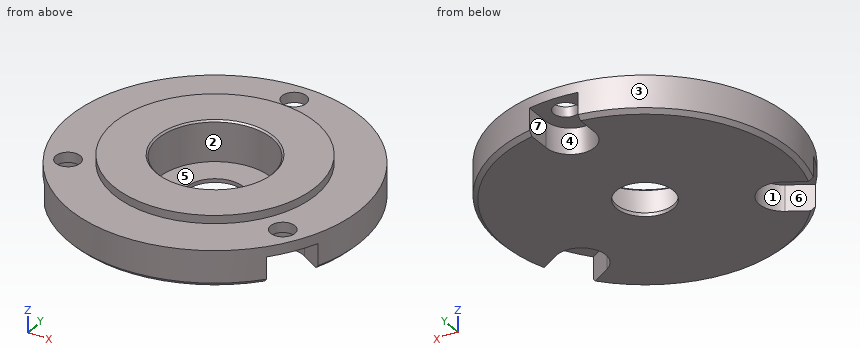
from build123d import *

# Parameters (mm, degrees)
ESQUISSE1_R             = 17.97
BOSS_EXTRU_1_DEPTH      = 4.45
ESQUISSE2_R             = 12.45
BOSS_EXTRU_2_DEPTH      = 1
CHANFREIN1_SIZE         = 0.5
ESQUISSE5_R             = 1.5
ENL_V_MAT_EXTRU_1_DEPTH = 6.45
ESQUISSE6_R             = 3.5
ENL_V_MAT_EXTRU_2_DEPTH = 6.45
ESQUISSE7_R             = 7
ENL_V_MAT_EXTRU_3_DEPTH = 5
ENL_V_MAT_EXTRU_4_DEPTH = 3.2
CHANFREIN2_SIZE         = 0.2


with BuildPart() as part:
    # Esquisse1 → Boss.-Extru.1 (new body)
    with BuildSketch(Plane.XY):
        with Locations((-74.842203198, 51.872077922)):
            Circle(ESQUISSE1_R)
    extrude(amount=BOSS_EXTRU_1_DEPTH)

    # Esquisse2 → Boss.-Extru.2 (add)
    with BuildSketch(Plane.XY.offset(4.45)):
        with Locations((-74.842203198, 51.872077922)):
            Circle(ESQUISSE2_R)
    extrude(amount=BOSS_EXTRU_2_DEPTH)

    # Chanfrein1
    chanfrein1_edges = [part.edges().sort_by_distance(p)[0] for p in [
        (-92.812203198, 51.872077922, 0),
    ]]
    chamfer(chanfrein1_edges, length=CHANFREIN1_SIZE)

    # Esquisse5 → Enlèv. mat.-Extru.1 (cut, through all)
    with BuildSketch(Plane(origin=(0, 0, 0), x_dir=(-1, 0, 0), z_dir=(0, 0, -1))):
        with Locations((74.842203198, 67.242077922)):
            Circle(ESQUISSE5_R)
        with Locations((61.531392742, 44.187077922)):
            Circle(ESQUISSE5_R)
        with Locations((88.153013654, 44.187077922)):
            Circle(ESQUISSE5_R)
    extrude(amount=-ENL_V_MAT_EXTRU_1_DEPTH, mode=Mode.SUBTRACT)

    # Esquisse6 → Enlèv. mat.-Extru.2 (cut, through all)
    with BuildSketch(Plane(origin=(0, 0, 0), x_dir=(-1, 0, 0), z_dir=(0, 0, -1))):
        with Locations((74.842203198, 51.872077922)):
            Circle(ESQUISSE6_R)
    extrude(amount=-ENL_V_MAT_EXTRU_2_DEPTH, mode=Mode.SUBTRACT)

    # Esquisse7 → Enlèv. mat.-Extru.3 (cut)
    with BuildSketch(Plane.XY.offset(5.45)):
        with Locations((-74.842203198, 51.872077922)):
            Circle(ESQUISSE7_R)
    extrude(amount=-ENL_V_MAT_EXTRU_3_DEPTH, mode=Mode.SUBTRACT)

    # Esquisse8 → Enlèv. mat.-Extru.4 (cut)
    with BuildSketch(Plane(origin=(0, 0, 0), x_dir=(-1, 0, 0), z_dir=(0, 0, -1))):
        with BuildLine():
            Line((71.842203198, 70.411905134), (71.842203198, 66.363654544))
            ThreePointArc((71.842203198, 66.363654544), (74.842203198, 63.363654544), (77.842203198, 66.363654544))
            Line((77.842203198, 66.363654544), (77.842203198, 70.411905134))
            Line((77.842203198, 70.411905134), (71.842203198, 70.411905134))
        make_face()
        with BuildLine():
            Line((60.379554388, 39.925212907), (63.849582418, 42.010216097))
            ThreePointArc((63.849582418, 42.010216097), (64.875970095, 46.126832224), (60.759353968, 47.153219901))
            Line((60.759353968, 47.153219901), (57.289325938, 45.068216711))
            Line((57.289325938, 45.068216711), (60.379554388, 39.925212907))
        make_face()
        with BuildLine():
            Line((92.371338943, 45.133431645), (88.865451092, 47.15755694))
            ThreePointArc((88.865451092, 47.15755694), (84.76737488, 46.059480728), (85.865451092, 41.961404517))
            Line((85.865451092, 41.961404517), (89.371338943, 39.937279222))
            Line((89.371338943, 39.937279222), (92.371338943, 45.133431645))
        make_face()
    extrude(amount=-ENL_V_MAT_EXTRU_4_DEPTH, mode=Mode.SUBTRACT)

    # Chanfrein2
    chanfrein2_edges = [part.edges().sort_by_distance(p)[0] for p in [
        (-81.842203198, 51.872077922, 5.45),
    ]]
    chamfer(chanfrein2_edges, length=CHANFREIN2_SIZE)


solid = part.part
Verification items for the finished model (mm, model axes). Face numbers are marked on the shaded views. A direction names the side the tool comes from. Give positions to 0.01 mm unless a question says otherwise; leave off trailing zeros. Write each loop counter-clockwise with the first axis right and the second up, starting at its lowest first coordinate (ties: lowest second). Pieces come first, ordered by that corner, then holes. Notation, with made-up numbers: M 53,-11 L 91,-11 A17 cw 91,8 Z; hole C 46.25,49.5 d7. An arc over 180 degrees is marked long. Write item = value, one per line.
(1) Draft check along Y on the marked faces 4, 5, 6 and 7. Enter one of: released by +Y, released by -Y, zero draft, split by the parting line, or undercut.
Found:
face_4 = released by +Y
face_5 = undercut
face_6 = undercut
face_7 = zero draft
(2) Sectioned sample at A-A (z = 1.05). Record the cut outline in (x, y), then the cut area to 3 significant figures.
Found:
outline = M -91.66,45.54 L -88.87,47.16 A3 cw -85.87,41.96 L -88.64,40.36 A17.97 ccw -61.06,40.34 L -63.85,42.01 A3 cw -60.76,47.15 L -58.03,45.52 A17.97 ccw -71.84,69.59 L -71.84,66.36 A3 cw -77.84,66.36 L -77.84,69.59 A17.97 ccw Z; hole C -74.84,51.87 d14
area = 757 mm2
(3) Access from +Z, -Z, +X, -X, +Y, -Y to the whole of each face (thin tool, end or side, straight path). Record for the marked faces 1, 2 and 3.
Found:
face_1 = -Z
face_2 = +Z
face_3 = +Z, -Z
(4) Material ranges on line 1 (Y direction, x = -73.5, z = 3.6); line 2 (X direction, y = 47, z = 2.15); line 3 (X direction, y = 44.5, z = 2.1), recorded low to high.
Found:
line_1 = 33.95 to 45, 58.74 to 66.57, 67.91 to 69.79
line_2 = -92.14 to -89.14, -85.62 to -79.87, -69.82 to -64.08, -60.5 to -57.55
line_3 = -84.37 to -65.3
(5) Go/stop test with flat-tipped pins: pin 1 Ø4 at (x, y) = (-88.5, 38) entering from +Z; pin 2 Ø2 at (x, y) = (-88.5, 43.5) entering from -Z; pin 3 Ø5 at (x, y) = (-75, 56.5) entering from +Z. Record where each tip stops, or that it passes through.
Found:
pin_1 = 4.45
pin_2 = 3.2
pin_3 = 5.38
